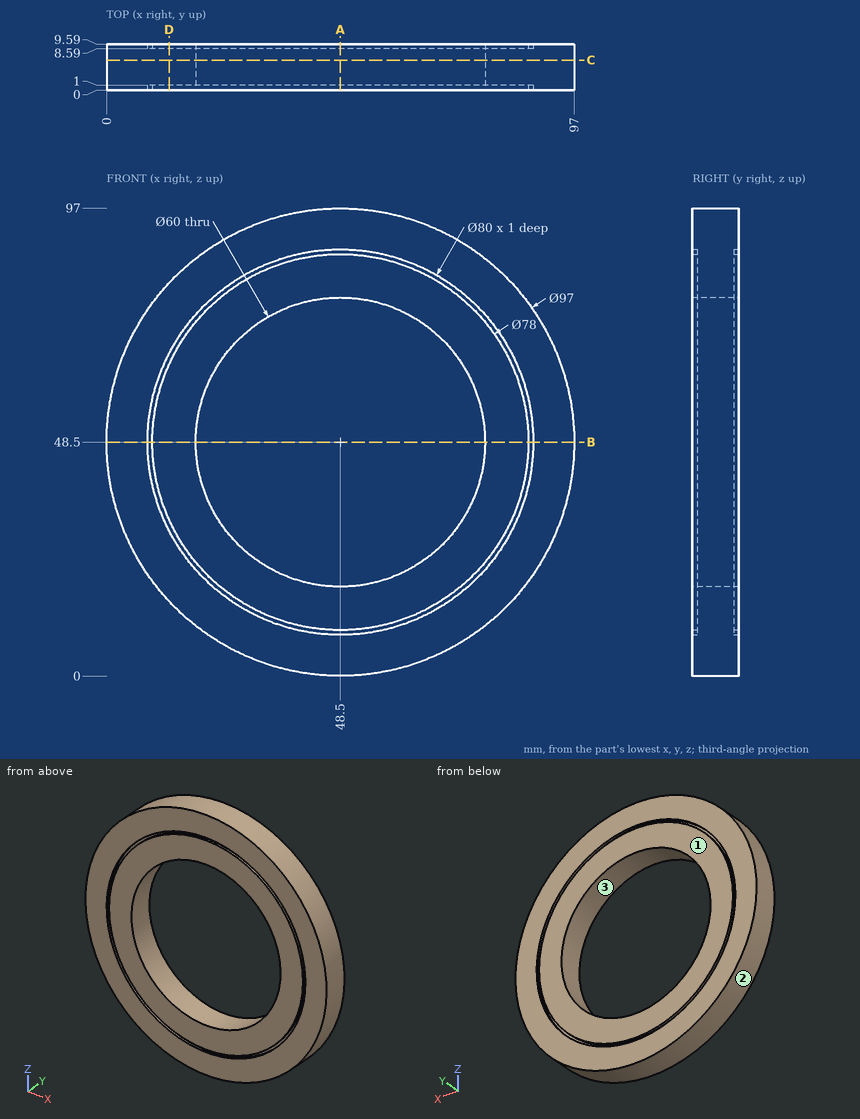
Verification items for this drawing (mm, ordinates from the low corner). Coordinates: 2 decimals unless noted, no trailing zeros. Order: outer loops, then holes, each group sorted by start corner. A loop starts at its lowest first (then second) coordinate and runs counter-clockwise, first axis right, second up. Notation, with made-up numbers: (3.25, 83) -> (44.25, 83) arc R25 cw to (44.25, 105) -> close; hole circle Ø11 at (65.5, 4.5). An arc over 180 degrees is marked (long way). Put each result on its own line as item: value. Start each with the question number.
1. Go/stop test with flat-tipped pins: pin 1 Ø3 at (y, z) = (6.5, 60) entering from -X; pin 2 Ø4 at (y, z) = (2.5, 41) entering from -X; pin 3 Ø1.5 at (y, z) = (3, 75) entering from +X. Record where each tip stops, or that it passes through.
2. Cross-section at C-C, the plane y = 6.25. Record the boundary of the cut face in (x, z).
3. Mould release check, pull along Z, two halves, no side actions. Record for the marked faces 1, 2 and 3: released by +Z, released by -Z, zero draft, split by the parting line, or undercut.
4. Cross-section at B-B, the plane z = 48.5. Record the boundary of the cut face in (x, y), then the cut area to 3 significant figures.
5. Cross-section at A-A, the plane x = 48.5. Record the boundary of the cut face in (y, z), then the cut area to 3 significant figures.
6. Material ranges on L1, parallel to X at y = 9.3, z = 48.5; L2, parallel to Z at x = 29.5, y = 4; L3, parallel to Z at x = 51, y = 3.5, recorded low to high. Write a range as [from, to].
7. Cross-section at D-D, the plane x = 13. Record the boundary of the cut face in (y, z), then the cut area to 3 significant figures.
Computed:
1. pin 1: x = 1.04
1. pin 2: x = 0.31
1. pin 3: x = 89.6
2. outline: circle Ø97 at (48.5, 48.5); hole circle Ø60 at (48.5, 48.5)
3. face 1: zero draft
3. face 2: split by the parting line
3. face 3: undercut
4. outline: (0, 0) -> (8.5, 0) -> (8.5, 1) -> (9.5, 1) -> (9.5, 0) -> (18.5, 0) -> (18.5, 9.59) -> (9.5, 9.59) -> (9.5, 8.59) -> (8.5, 8.59) -> (8.5, 9.59) -> (0, 9.59) -> close; (78.5, 0) -> (87.5, 0) -> (87.5, 1) -> (88.5, 1) -> (88.5, 0) -> (97, 0) -> (97, 9.59) -> (88.5, 9.59) -> (88.5, 8.59) -> (87.5, 8.59) -> (87.5, 9.59) -> (78.5, 9.59) -> close
4. area: 351 mm2
5. outline: (0, 0) -> (9.59, 0) -> (9.59, 8.5) -> (8.59, 8.5) -> (8.59, 9.5) -> (9.59, 9.5) -> (9.59, 18.5) -> (0, 18.5) -> (0, 9.5) -> (1, 9.5) -> (1, 8.5) -> (0, 8.5) -> close; (0, 78.5) -> (9.59, 78.5) -> (9.59, 87.5) -> (8.59, 87.5) -> (8.59, 88.5) -> (9.59, 88.5) -> (9.59, 97) -> (0, 97) -> (0, 88.5) -> (1, 88.5) -> (1, 87.5) -> (0, 87.5) -> close
5. area: 351 mm2
6. L1: [0, 8.5], [9.5, 18.5], [78.5, 87.5], [88.5, 97]
6. L2: [3.88, 25.28], [71.72, 93.12]
6. L3: [0.06, 18.6], [78.4, 96.94]
7. outline: (0, 15.45) -> (9.59, 15.45) -> (9.59, 30.07) -> (8.59, 30.07) -> (8.59, 32.35) -> (9.59, 32.35) -> (9.59, 64.65) -> (8.59, 64.65) -> (8.59, 66.93) -> (9.59, 66.93) -> (9.59, 81.55) -> (0, 81.55) -> (0, 66.93) -> (1, 66.93) -> (1, 64.65) -> (0, 64.65) -> (0, 32.35) -> (1, 32.35) -> (1, 30.07) -> (0, 30.07) -> close
7. area: 625 mm2
